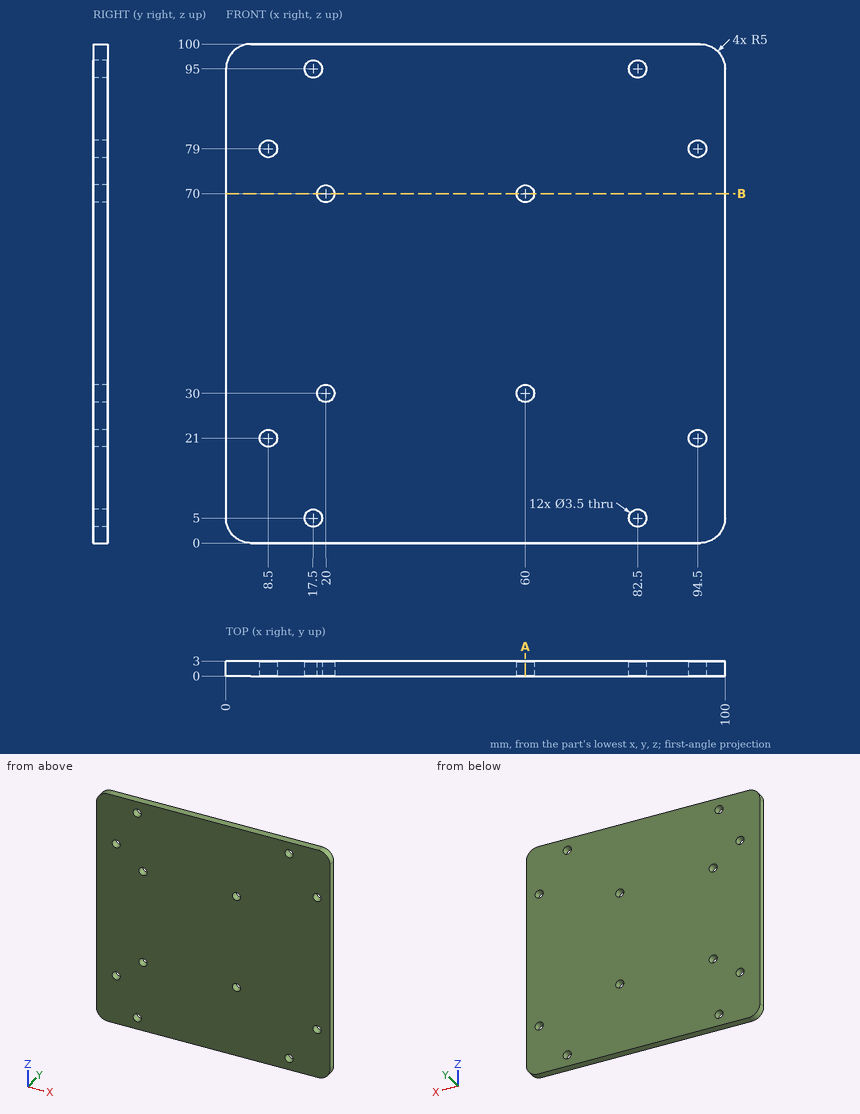
Part print with two shaded views. Sizes in mm from the minimum x, y, z corner. Round coordinates to 2 decimals unless told otherwise and drop trailing zeros. Order: outer loops, then holes, each group sorted by start corner. A loop starts at its lowest first (then second) coordinate and runs counter-clockwise, first axis right, second up. Notation, with made-up numbers: M -26,37.25 L 14,37.25 A25 cw 14,73.25 Z; hole C 61.5,73 d9. An arc over 180 degrees is marked long. Answer in a Markdown table with one row per item. Add a question column.
Q1. Wall check: L1, parallel to X at y = 1.9, z = 79; L2, parallel to Z at x = 8.5, y = 1.7; L3, parallel to X at y = 1.45, z = 95. Give the ranges that are in metal, low to high. Write a range as from..to.
Q2. Cut at A-A on x = 60. Give the cut face in (y, z).
Q3. Cut at B-B on z = 70. Give the cut face in (x, y).
Established:
| question | item | result |
|---|---|---|
| 1 | L1 | x = 0..6.75, 10.25..92.75, 96.25..100 |
| 1 | L2 | z = 0..19.25, 22.75..77.25, 80.75..100 |
| 1 | L3 | x = 0..15.75, 19.25..80.75, 84.25..100 |
| 2 | outline | M 0,0 L 3,0 L 3,28.25 L 0,28.25 Z; M 0,31.75 L 3,31.75 L 3,68.25 L 0,68.25 Z; M 0,71.75 L 3,71.75 L 3,100 L 0,100 Z |
| 3 | outline | M 0,0 L 18.25,0 L 18.25,3 L 0,3 Z; M 21.75,0 L 58.25,0 L 58.25,3 L 21.75,3 Z; M 61.75,0 L 100,0 L 100,3 L 61.75,3 Z |
